Source: CAD feature listing. Evaluate the final solid. Frame: model axes, mm. Coordinates: 2 decimals unless noted, no trailing zeros. Order: outer loops, then holes, each group sorted by start corner. A loop starts at its lowest first (then second) coordinate and runs counter-clockwise, first axis right, second up. Notation, with made-up numbers: (-37, 11.5) -> (18, 11.5) arc R4 cw to (18, 15.5) -> close; hole circle Ø9 at (5.25, 65). An arc over 180 degrees is marked (long way). Put each result on its own line as item: value.
Autodesk Inventor part; units mm, degrees
ref_plane "YZ Plane" through (0, 0, 0) normal (1, 0, 0) x (0, 1, 0)
ref_plane "XZ Plane" through (0, 0, 0) normal (0, 1, 0) x (-1, 0, 0)
ref_plane "XY Plane" through (0, 0, 0) normal (0, 0, 1) x (1, 0, 0)
sketch "Sketch1" plane through (0, 0, 0) normal (0, 0, 1) x (1, 0, 0)
  line L0 (0, 0) -> (254, 0)
  circle A0 centre (127, 20.32) radius 9.652 construction
  line L1 (127, 38.1) -> (127, 0) construction
  arc A1 (85.2807, 20.21) -> (113.8319, 32.6419) centre (83.7743, 62.6708) ccw
  arc A2 (127, 38.1) -> (113.8319, 32.6419) centre (127, 19.4864) ccw
  arc A3 (140.1681, 32.6419) -> (168.7193, 20.21) centre (170.2257, 62.6708) ccw
  arc A4 (140.1681, 32.6419) -> (127, 38.1) centre (127, 19.4864) ccw
  line L2 (85.2807, 20.21) -> (19.2407, 20.21)
  line L3 (168.7193, 20.21) -> (234.7593, 20.21)
  arc A5 (254, 0) -> (234.7593, 20.21) centre (234.7593, 0.9461) ccw
  arc A6 (19.2407, 20.21) -> (0, 0) centre (21.9577, -1.6406) ccw
  dimension "d2" = 19.304
  dimension "d74" = 254
  dimension "d75" = 20.32
  dimension "d76" = 38.1
  dimension "d78" = 42.4876
  dimension "d79" = 18.6136
  dimension "d89" = 66.04
  dimension "d90" = 66.04
  dimension "d91" = 22.0189
  dimension "d92" = 19.2639
  dimension "d93" = 21.8506
extrude "Extrusion2" add sketch "Sketch1" along normal blind 6.35
sketch "Sketch5" plane through (0, 0, 6.35) normal (0, 0, 1) x (1, 0, 0)
  circle A0 centre (127, 19.05) radius 9.652
  line L0 (0, 0) -> (254, 0)
  arc A1 (140.1681, 32.6419) -> (113.8319, 32.6419) centre (127, 19.4864) ccw
  point P0 (127, 1.27)
  point P1 (127, 38.1)
  dimension "d58" = 19.304
  dimension "d87" = 19.05
hole "Hole3" at (127, 19.05, 6.35) direction (0, 0, -1) diameter 2.54 end through all
properties part number "holder"
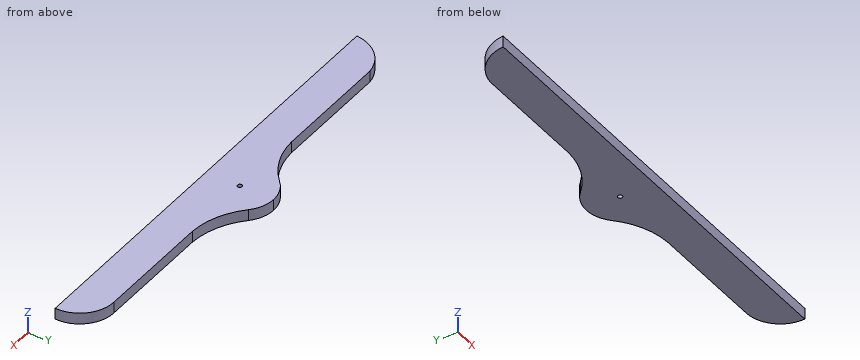
1. Cut plane B-B on x = 71. Output: boundary loops of the cut face in (y, z), plus the area to 3 significant figures.
Numbers:
outline: (0, 0) -> (20.21, 0) -> (20.21, 6.35) -> (0, 6.35) -> close
area: 128 mm2
2. Ray query, line 1 along Y through (x, z) = (127, 4); line 2 along Y through (x, z) = (205.5, 3.25); line 3 along Y through (x, z) = (147.5, 4.5). Return the intervals inside material, ascending.
Numbers:
line 1: y = 0 to 17.78, 20.32 to 38.1
line 2: y = 0 to 20.21
line 3: y = 0 to 26.77
3. Cut plane A-A on z = 3. Output: boundary loops of the cut face in (x, y).
Numbers:
outline: (0, 0) -> (254, 0) arc R19.26 ccw to (234.76, 20.21) -> (168.72, 20.21) arc R42.49 cw to (140.17, 32.64) arc R18.61 ccw to (127, 38.1) arc R18.61 ccw to (113.83, 32.64) arc R42.49 cw to (85.28, 20.21) -> (19.24, 20.21) arc R22.02 ccw to start; hole circle Ø2.54 at (127, 19.05)
4. First-contact query: pin 1 (1.5 mm diameter, centred on y = 16.5, z = 4, fed in from -X). Flat tip, straight axial feed; report the tip coordinate or a pass-through.
Numbers:
pin 1: stops at x = 8.45
5. Cut plane C-C on y = 23. Output: boundary loops of the cut face in (x, z).
Numbers:
outline: (98.99, 0) -> (155.01, 0) -> (155.01, 6.35) -> (98.99, 6.35) -> close
